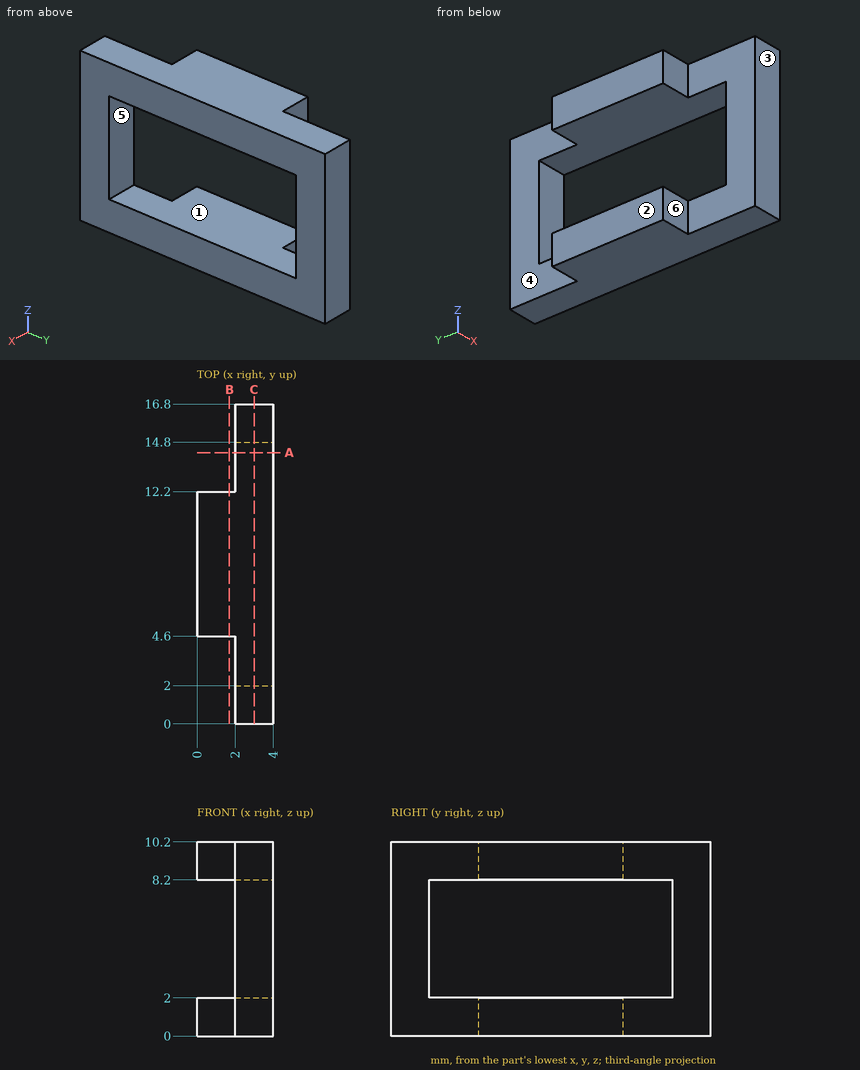
Here's the drawing with two shaded views (mm, measured from the low corner). I have some questions. A direction names the side the tool comes from. Coordinates: 2 decimals unless noted, no trailing zeros. Order: outer loops, then holes, each group sorted by start corner. A loop starts at its lowest first (then second) coordinate and runs counter-clockwise, first axis right, second up. Notation, with made-up numbers: M 88.5,19 L 106.5,19 A35 cw 106.5,53 Z; hole C 40.25,78 d3. An arc over 180 degrees is marked long. Write item = value, one per line.
(1) Suppose I cut it at B-B on x = 1.7. Please give me the cut outline in (y, z).
Results are:
outline = M 4.6,0 L 12.2,0 L 12.2,2 L 4.6,2 Z; M 4.6,8.2 L 12.2,8.2 L 12.2,10.2 L 4.6,10.2 Z
(2) Suppose I cut it at C-C on x = 3. Please give me the cut outline in (y, z).
Results are:
outline = M 0,0 L 16.8,0 L 16.8,10.2 L 0,10.2 Z; hole M 2,2 L 14.8,2 L 14.8,8.2 L 2,8.2 Z
(3) I need wall thicknesses on line 1 along Z through (x, y) = (2.8, 5.5); line 2 along Y through (x, z) = (2.3, 6.25); line 3 along X through (y, z) = (2.75, 1). Which ranges of each line are inside material? Lowest first, please. Write a range as [from, to].
Results are:
line_1 = [0, 2], [8.2, 10.2]
line_2 = [0, 2], [14.8, 16.8]
line_3 = [2, 4]
(4) For the marked faces 4, 5 and 6, which set-ups out of +Z, -Z, +X, -X, +Y, -Y let a thin tool reach every point of the face, with its end or its side?
Results are:
face_4 = +Z, -Z, -X, +Y
face_5 = +X, -X
face_6 = +Z, -Z, -X, -Y
(5) For pin 1 Ø2.5 at (y, z) = (2.5, 2.5) entering from -X; pin 2 Ø0.6 at (x, z) = (1, 1) entering from -Y; pin 3 Ø0.6 at (x, z) = (1, 9.5) entering from +Y, each with a flat end and sliding along its axis, tell me the tip position at first contact or that it passes through.
Results are:
pin_1 = 2
pin_2 = 4.6
pin_3 = 12.2
(6) If we mould it in two halves opening along Y, with no side actions, what happens to the marked faces 1, 2 and 3? For each: pulls with the +Y half, pulls with the -Y half, needs draft (parallel to the pull), parting line crosses it, or undercut.
Results are:
face_1 = undercut
face_2 = needs draft
face_3 = pulls with the -Y half
(7) Suppose I cut it at A-A on y = 14.25. Please give me the cut outline in (x, z), plus the area to 3 significant figures.
Results are:
outline = M 2,0 L 4,0 L 4,2 L 2,2 Z; M 2,8.2 L 4,8.2 L 4,10.2 L 2,10.2 Z
area = 8.00 mm2
